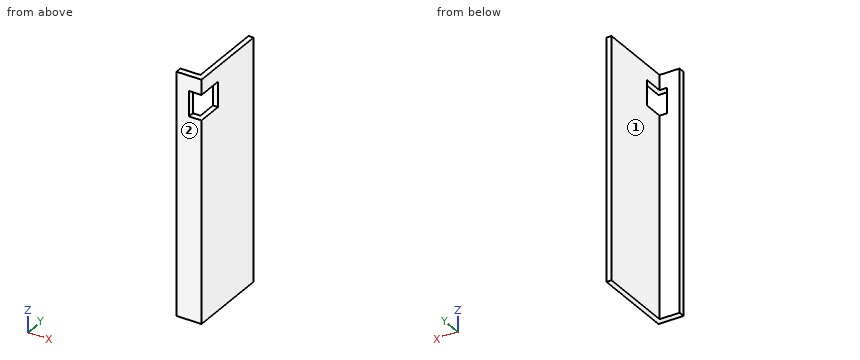
from build123d import *

# Parameters (mm, degrees)
F0_W     = 838.2
F0_H     = 2438.4
F1_DEPTH = 50.8
F2_W     = 63.5
F2_H     = 2438.4
F3_DEPTH = 203.2
F5_W     = 304.8
F5_H     = 254
F6_DEPTH = 127


with BuildPart() as f1:
    # F0 (on Right) → F1 (new body)
    with BuildSketch(Plane.YZ):
        Rectangle(F0_W, F0_H)
    extrude(amount=F1_DEPTH)

    # F2 (on face) → F3 (join)
    with BuildSketch(Plane(origin=(0, 0, 0), x_dir=(0, -1, 0), z_dir=(-1, 0, 0))):
        with Locations((387.35, 0)):
            Rectangle(F2_W, F2_H)
    extrude(amount=F3_DEPTH)

    # F5 (on face) → F6 (cut)
    with BuildSketch(Plane.YZ.offset(50.8)):
        with Locations((-304.8, 939.8)):
            Rectangle(F5_W, F5_H)
    extrude(amount=-F6_DEPTH, mode=Mode.SUBTRACT)


solid = f1.part
Could you check a few things on this model? Use its own coordinates, in mm. Face numbers are marked on the shaded views. A direction names the side the tool comes from. Give positions to 0.01 mm unless a question says otherwise; leave off trailing zeros. Loops run counter-clockwise (first coordinate to the right, second up) from the corner with the lowest first, then second, coordinate; pieces in that order, holes last. Notation, with made-up numbers: (15.5, 11.5) -> (23.5, 11.5) arc R21 cw to (23.5, 46.5) -> close; hole circle Ø10 at (2, 26). An arc over 180 degrees is marked (long way). Return JSON: item names as keys, results as strings.
Item 1: If we section it at B-B on x = -37: List the corners of the cut face in (y, z) for me.
Geometry results:
{"outline": "(-419.1, -1219.2) -> (-355.6, -1219.2) -> (-355.6, 812.8) -> (-419.1, 812.8) -> close; (-419.1, 1066.8) -> (-355.6, 1066.8) -> (-355.6, 1219.2) -> (-419.1, 1219.2) -> close"}
Item 2: If we section it at A-A on y = -210: List the corners of the cut face in (x, z) for me.
Geometry results:
{"outline": "(0, -1219.2) -> (50.8, -1219.2) -> (50.8, 812.8) -> (0, 812.8) -> close; (0, 1066.8) -> (50.8, 1066.8) -> (50.8, 1219.2) -> (0, 1219.2) -> close"}
Item 3: Which directions (+Z, -Z, +X, -X, +Y, -Y) give clear straight access to the entire face, cutting with the end or side of a thin tool? Please do the marked faces 1 and 2.
Geometry results:
{"face 1": "+Z, -Z, -X, +Y", "face 2": "+Z, -Z, +X, -X, -Y"}
Item 4: I'm going to push flat-ended pins straight in: pin 1 (6 mm diameter, centred on y = -83.5, z = -115, fed in from -X); pin 2 (6 mm diameter, centred on x = -46, z = -287, fed in from +Y); pin 3 (15 mm diameter, centred on x = 29, z = 996.5, fed in from -Y). Where does each tip first touch, or does it pass through?
Geometry results:
{"pin 1": "stops at x = 0", "pin 2": "stops at y = -355.6", "pin 3": "stops at y = -152.4"}
Item 5: If we section it at C-C on z = 717: List the corners of the cut face in (x, y) for me, plus the area to 3 significant figures.
Geometry results:
{"outline": "(-203.2, -419.1) -> (50.8, -419.1) -> (50.8, 419.1) -> (0, 419.1) -> (0, -355.6) -> (-203.2, -355.6) -> close", "area": "55,500 mm²"}
Item 6: If we section it at D-D on x = -163: List the corners of the cut face in (y, z) for me.
Geometry results:
{"outline": "(-419.1, -1219.2) -> (-355.6, -1219.2) -> (-355.6, 1219.2) -> (-419.1, 1219.2) -> close"}
Item 7: I need wall thicknesses on L1, parallel to Z at x = -72.5, y = -375; L2, parallel to Y at x = -92, z = -261; L3, parallel to X at y = -206.5, z = -290. Which ranges of each line are inside material? Lowest first, please. Write a range as from..to.
Geometry results:
{"L1": "z = -1219.2..812.8, 1066.8..1219.2", "L2": "y = -419.1..-355.6", "L3": "x = 0..50.8"}
